Autodesk Inventor part; units mm, degrees
ref_plane "YZ Plane" through (0, 0, 0) normal (1, 0, 0) x (0, 1, 0)
ref_plane "XZ Plane" through (0, 0, 0) normal (0, 1, 0) x (-1, 0, 0)
ref_plane "XY Plane" through (0, 0, 0) normal (0, 0, 1) x (1, 0, 0)
sketch "Sketch1" plane through (0, 0, 0) normal (0, 0, 1) x (1, 0, 0)
  line L0 (0, 0) -> (13.0048, 0)
  line L1 (13.0048, 0) -> (13.0048, 13.0048)
  line L2 (13.0048, 13.0048) -> (0, 13.0048)
  line L3 (0, 13.0048) -> (0, 0)
  dimension "d0" = 13.0048
  dimension "d1" = 13.0048
extrude "Extrusion1" add sketch "Sketch1" along normal blind 6.5
sketch "Sketch2" plane through (0, 0, 6.5) normal (0, 0, 1) x (1, 0, 0)
  circle A0 centre (6.5024, 6.5024) radius 2.65
  line L0 (13.0048, 0) -> (13.0048, 13.0048)
  line L1 (13.0048, 13.0048) -> (0, 13.0048)
  point P0 (0, 0)
  point P1 (13.0048, 6.5024)
  point P2 (6.5024, 13.0048)
  dimension "d4" = 5.3
extrude "Extrusion2" add sketch "Sketch2" along normal blind 2.6
fillet "Fillet1" radius 0.508 1 edges at (3.8524, 6.5024, 9.1)
properties part number "Power switch"
Geometry: final body of the model. Coordinates: model frame, mm. A direction names the side the tool comes from. Coordinates: 2 decimals unless noted, no trailing zeros. Order: outer loops, then holes, each group sorted by start corner. A loop starts at its lowest first (then second) coordinate and runs counter-clockwise, first axis right, second up.
(1) Material intervals for probe 1 along Z at (x, y) = (11, 4.5); probe 2 along Y at (x, z) = (5.75, 6.75); probe 3 along Z at (x, y) = (6.5, 4), sorted ascending.
(2) Access query for faces 1 (the face through (4.55, 4.71, 7.53)), 2 (the face through (13.005, 6, 3)). Directions: +Z, -Z, +X, -X, +Y, -Y. A direction counts if a zero-diameter tool reaches every point of the face in a straight line with its end or side. Return the directions, or none.
(3) Section query A-A (y = 1.25). Return the cut outline in (x, z), plus the area to 3 significant figures.
Solution:
1. probe 1: z = 0 to 6.5
1. probe 2: y = 3.96 to 9.04
1. probe 3: z = 0 to 8.95
2. face 1: +Z
2. face 2: +Z, -Z, +X, +Y, -Y
3. outline: (0, 0) - (13, 0) - (13, 6.5) - (0, 6.5) - close
3. area: 84.5 mm2
